```python
from build123d import *

# Parameters (mm, degrees)
F1_DEPTH  = 19.05
F3_DEPTH  = 6.35
F4_R      = 0.635
F5_DEPTH  = 1.5691231
F6_R      = 2.53999
F7_R      = 0.635
F9_DEPTH  = 6.35
F11_D     = 2.54
F16_D     = 127
F16_DEPTH = 15.876


# Not quite as in the source:
# - a fillet or chamfer is up to 0.001 mm smaller than in the source, because OpenCascade refuses the exact size
# - a length typed as a fraction of an inch, garbled in the dataset ("3 / 203.2 mm" for 3/8 in), is restored
# - the program builds the solid bodies; features that only make, move or delete a surface that nothing else refers to are left out


with BuildPart() as f1:
    # F0 (on Top) → F1 (new body)
    with BuildSketch(Plane.XY):
        Polygon((6.6501818182, 11.43), (0, 11.43), (-6.6501818182, 11.43), (-13.9976640991, 4.0825177191), (-13.9976640991, 0), (-13.9976640991, -4.0825177191), (-6.6501818182, -11.43), (0, -11.43), (6.6501818182, -11.43), (13.9976640991, -4.0825177191), (13.9976640991, 0), (13.9976640991, 4.0825177191), align=None)
        with BuildLine():
            ThreePointArc((6.5717879374, 9.3518181818), (10.1429886159, 5.26922024), (11.43, 0))
            ThreePointArc((11.43, 0), (10.1429886159, -5.26922024), (6.5717879374, -9.3518181818))
            Line((6.5717879374, -9.3518181818), (0, -9.3518181818))
            Line((0, -9.3518181818), (-6.5717879374, -9.3518181818))
            ThreePointArc((-6.5717879374, -9.3518181818), (-10.1429886159, -5.26922024), (-11.43, 0))
            ThreePointArc((-11.43, 0), (-10.1429886159, 5.26922024), (-6.5717879374, 9.3518181818))
            Line((-6.5717879374, 9.3518181818), (0, 9.3518181818))
            Line((0, 9.3518181818), (6.5717879374, 9.3518181818))
        make_face(mode=Mode.SUBTRACT)
    extrude(amount=F1_DEPTH)

    # F2 (on Top) → F3 (join)
    with BuildSketch(Plane.XY):
        Polygon((12.9991231, -2.54), (12.9991231, 0), (12.9991231, 2.54), (11.43, 2.54), (11.43, 0), (11.43, -2.54), align=None)
    extrude(amount=-F3_DEPTH)

    # F4 (on face) → F5 (join)
    with BuildSketch(Plane.YZ.offset(12.9991231)):
        with Locations((0, -5.08)):
            Circle(F4_R)
    extrude(amount=F5_DEPTH)

    # F6 (radius 2.54 in the source; OpenCascade refuses exactly that, so slightly less here)
    f6_edges = [f1.edges().sort_by_distance(p)[0] for p in [
        (12.214562, -2.54, -6.35),
        (12.214562, 2.54, -6.35),
    ]]
    fillet(f6_edges, radius=F6_R)

    # F7
    f7_edges = [f1.edges().sort_by_distance(p)[0] for p in [
        (14.568246, -0.635, -5.08),
    ]]
    fillet(f7_edges, radius=F7_R)

    # F8 (on face) → F9 (join)
    with BuildSketch(Plane.XY.offset(19.05)):
        Polygon((13.9976640991, 2.54), (12.4285360385, 2.54), (12.4285360385, 0), (12.4285360385, -2.54), (13.9976640991, -2.54), (13.9976640991, 0), align=None)
    extrude(amount=F9_DEPTH)

    # F11 (through all)
    with Locations(Plane.YZ.offset(13.9976640991)):
        with Locations((0, 22.86)):
            Hole(F11_D / 2)

    # F12: F1 across plane


with BuildPart() as f1_1:
    add(f1.part)
    add(f1.part.mirror(Plane.YZ))

    # F16 (through all, one way)
    with BuildSketch(Plane(origin=(0, 0, 9.525), x_dir=(1, 0, 0), z_dir=(0, 0, -1))):
        with Locations((0, 0)):
            Circle(F16_D / 2)
    extrude(amount=-F16_DEPTH, mode=Mode.SUBTRACT)


solid = f1_1.part
```
Verification items for the finished model (mm, model axes). A direction names the side the tool comes from. Coordinates: 2 decimals unless noted, no trailing zeros. Loops run counter-clockwise (first coordinate to the right, second up) from the corner with the lowest first, then second, coordinate; pieces in that order, holes last. Notation, with made-up numbers: (8.25, 10.5) - (39.25, 10.5) arc R13 cw to (39.25, 25.5) - close; hole circle Ø3 at (87, -29.75). An arc over 180 degrees is marked (long way). Put each result on its own line as item: value.
Item 1: Draft check along Y on faces 6 (the face through (13.998, 0, 5)), 7 (the face through (11.43, 0.15, 4.7)), 8 (the face through (-10.27, 7.81, 4.7)), 9 (the face through (-13.46, -0.08, -4.45)). Enter one of: pulls with the +Y half, pulls with the -Y half, needs draft (parallel to the pull), parting line crosses it, or undercut.
Conclusion:
face 6: needs draft
face 7: undercut
face 8: pulls with the +Y half
face 9: parting line crosses it
Item 2: Section check C-C (y = 5). Enter the section's corners in (x, z) (3 decimals).
Conclusion:
outline: (-13.08, 0) - (-10.278, 0) - (-10.278, 9.525) - (-13.08, 9.525) - close; (10.278, 0) - (13.08, 0) - (13.08, 9.525) - (10.278, 9.525) - close
Item 3: Section check B-B (z = 7.5). Enter the section's corners in (x, y), then the cut area to 3 significant figures.
Conclusion:
outline: (-14, -4.08) - (-6.65, -11.43) - (6.65, -11.43) - (14, -4.08) - (14, 4.08) - (6.65, 11.43) - (-6.65, 11.43) - (-14, 4.08) - close; hole (-6.57, -9.35) - (6.57, -9.35) arc R11.43 ccw to (6.57, 9.35) - (-6.57, 9.35) arc R11.43 ccw to start
area: 159 mm2
Item 4: Section check D-D (z = -5.08). Enter the section's corners in (x, y) (3 decimals).
Conclusion:
outline: (-13.933, -0.635) - (-12.999, -0.635) - (-12.999, -2.2) - (-11.43, -2.2) - (-11.43, 2.2) - (-12.999, 2.2) - (-12.999, 0.635) - (-13.933, 0.635) arc R0.635 ccw to start; (11.43, -2.2) - (12.999, -2.2) - (12.999, -0.635) - (13.933, -0.635) arc R0.635 ccw to (13.933, 0.635) - (12.999, 0.635) - (12.999, 2.2) - (11.43, 2.2) - close
Item 5: Section check A-A (x = -5.5). Enter the section's corners in (y, z) (3 decimals).
Conclusion:
outline: (-11.43, 0) - (-9.352, 0) - (-9.352, 9.525) - (-11.43, 9.525) - close; (9.352, 0) - (11.43, 0) - (11.43, 9.525) - (9.352, 9.525) - close
Item 6: Scan lines: line 1 along Y through (x, z) = (-5.75, 8.25); line 2 along X through (y, z) = (1, -0.25); line 3 along Z through (x, y) = (-6.5, 9.75) (3 decimals). Record each from-to range of solid material in increasing order.
Conclusion:
line 1: y = -11.43 to -9.35, 9.35 to 11.43
line 2: x = -13 to -11.43, 11.43 to 13
line 3: z = 0 to 9.525
Item 7: Gauge pin test, flat ends, axial feed: pin 1 Ø4 at (y, z) = (-4, -4) entering from +X; pin 2 Ø4 at (y, z) = (4.5, 0.5) entering from +X; pin 3 Ø0.8 at (x, z) = (-12, -2) entering from +Y; pin 4 Ø4 at (x, y) = (-5, -6.5) entering from -Z. Record the tip position at first contact, or that the pin passes through.
Conclusion:
pin 1: stops at x = 13
pin 2: stops at x = 14
pin 3: stops at y = 2.54
pin 4: passes through
Item 8: Set-up check for faces 1 (the face through (-11.43, 0, -3)), 2 (the face through (-11.43, -0.15, 4.7)), 3 (the face through (-12, 2.54, -2)), 4 (the face through (10.27, -7.81, 4.7)), 5 (the face through (12, -2.54, -2)): record each of +Z, -Z, +X, -X, +Y, -Y from which the full face is reachable in a straight line by a thin tool's end or side.
Conclusion:
face 1: -Z, +Y, -Y
face 2: +Z, -Z
face 3: -Z, +X, -X, +Y
face 4: +Z, -Z, +X, -Y
face 5: -Z, +X, -X, -Y
